Input: part model. Units: mm. Frame: model coordinates. Round coordinates to 2 decimals unless told otherwise and drop trailing zeros. Order: outer loops, then holes, each group sorted by start corner. A loop starts at its lowest first (then second) coordinate and runs counter-clockwise, first axis right, second up. Notation, with made-up numbers: (71.25, 2) -> (97.25, 2) arc R10 cw to (97.25, 18) -> close; hole circle Ø8 at (65.25, 24.25). An arc over 180 degrees is marked (long way). Use a Markdown table: item, result.
from build123d import *

# Parameters (mm, degrees)
F0_W           = 32
F0_H           = 32
F0_R           = 2
F0_R_2         = 1.1
F0_R_3         = 7
F1_DEPTH       = 1.5875
F3_D           = 4
F3_CSINK_D     = 8
F3_CSINK_ANGLE = 90
F4_D           = 2
F4_CSINK_D     = 4
F4_CSINK_ANGLE = 90
F5_R           = 4


with BuildPart() as f1:
    # F0 (on Right) → F1 (new body)
    with BuildSketch(Plane.YZ):
        Rectangle(F0_W, F0_H)
        with Locations((-11.313708, -11.313708)):
            Circle(F0_R, mode=Mode.SUBTRACT)
        with Locations((0, -9)):
            Circle(F0_R_2, mode=Mode.SUBTRACT)
        with Locations((11.313708, -11.313708)):
            Circle(F0_R, mode=Mode.SUBTRACT)
        with Locations((-9, 0)):
            Circle(F0_R_2, mode=Mode.SUBTRACT)
        with Locations((-11.313708, 11.313708)):
            Circle(F0_R, mode=Mode.SUBTRACT)
        Circle(F0_R_3, mode=Mode.SUBTRACT)
        with Locations((9, 0)):
            Circle(F0_R_2, mode=Mode.SUBTRACT)
        with Locations((0, 9)):
            Circle(F0_R_2, mode=Mode.SUBTRACT)
        with Locations((11.313708, 11.313708)):
            Circle(F0_R, mode=Mode.SUBTRACT)
    extrude(amount=F1_DEPTH)

    # F3 (through all)
    with Locations(Plane.YZ.offset(1.5875)):
        with Locations((-11.313708, 11.313708), (11.313708, 11.313708), (11.313708, -11.313708), (-11.313708, -11.313708)):
            CounterSinkHole(F3_D / 2, F3_CSINK_D / 2, counter_sink_angle=F3_CSINK_ANGLE)

    # F4 (through all)
    with Locations(Plane.YZ.offset(1.5875)):
        with Locations((-9, 0), (0, 9), (9, 0), (0, -9)):
            CounterSinkHole(F4_D / 2, F4_CSINK_D / 2, counter_sink_angle=F4_CSINK_ANGLE)

    # F5
    f5_edges = [f1.edges().sort_by_distance(p)[0] for p in [
        (0.79375, -16, 16),
        (0.79375, 16, 16),
        (0.79375, 16, -16),
        (0.79375, -16, -16),
    ]]
    fillet(f5_edges, radius=F5_R)


solid = f1.part
1) Line query: L1, parallel to Y at x = 0.25, z = 0; L2, parallel to Y at x = 1.5, z = -13; L3, parallel to Z at x = 1.1, y = 0. Output: solid intervals per line, ascending. Write a range as [from, to].
Results found:
| item | result |
|---|---|
| L1 | y = [-16, -10.1], [-7.9, -7], [7, 7.9], [10.1, 16] |
| L2 | y = [-15.87, -14.84], [-7.78, 7.78], [14.84, 15.87] |
| L3 | z = [-16, -10.51], [-7.49, -7], [7, 7.49], [10.51, 16] |
2) Cut plane B-B on z = -5. Return loops of the section in (x, y), and give its area (3 significant figures).
Results found:
| item | result |
|---|---|
| outline | (0, -16) -> (1.59, -16) -> (1.59, -4.9) -> (0, -4.9) -> close; (0, 4.9) -> (1.59, 4.9) -> (1.59, 16) -> (0, 16) -> close |
| area | 35.2 mm² |
3) Pull-direction query (Y, two-part tool) for faces 1 (the cylindrical face through (0.783, 6.466, -2.681)), 2 (the cylindrical face through (0.339, -0.238, -10.074)), 3 (the cylindrical face through (0.805, 14.859, -14.797)), 4 (the flat face through (1, 0, -16)); classes: +Y half, -Y half, draft (parallel to the pull), parting line (faces both ways), or undercut.
Results found:
| item | result |
|---|---|
| face 1 | undercut |
| face 2 | undercut |
| face 3 | +Y half |
| face 4 | draft |
4) Cut plane C-C on x = 1.25. Count the separate pieces of the cut face and the enclosed holes in it, and give its area (3 significant figures).
Results found:
| item | result |
|---|---|
| separate pieces | 1 |
| enclosed holes | 9 |
| area | 653 mm² |
5) Pin query (flat end, axial travel): pin 1 Ø3 at (y, z) = (-1, 7.5) entering from +X. Return the tip coordinate at first contact, or that it passes through.
Results found:
| item | result |
|---|---|
| pin 1 | stops at x = 1.59 |
6) Cut plane A-A on y = -4. Return loops of the section in (x, z), and give its area (3 significant figures).
Results found:
| item | result |
|---|---|
| outline | (0, -16) -> (1.59, -16) -> (1.59, -5.74) -> (0, -5.74) -> close; (0, 5.74) -> (1.59, 5.74) -> (1.59, 16) -> (0, 16) -> close |
| area | 32.6 mm² |
